Input: part model. Units: mm. Frame: model coordinates. A direction names the side the tool comes from. Coordinates: 2 decimals unless noted, no trailing zeros. Loops run counter-clockwise (first coordinate to the right, second up) from the corner with the lowest first, then second, coordinate; pieces in that order, holes last. Notation, with made-up numbers: (6, 15.5) -> (57, 15.5) arc R33 ccw to (57, 47.5) -> close; hole circle Ø1 at (69, 43). An arc over 180 degrees is marked (long way). Put each result on its own line as item: value. Start each with the question number.
1) Cut plane C-C (x = -8). Return the cut outline in (y, z).
2) Cut plane D-D (y = 4.25). Return the cut outline in (x, z).
3) Material intervals for L1, parallel to X at y = 3, z = 1.75; L2, parallel to Z at x = -19, y = -5.5; L3, parallel to Y at x = -22.5, z = -3.5, sorted ascending.
4) Set-up query: faces 1 (the flat face through (30, 0, 0)), 2 (the cylindrical face through (28, -3, 0)), 3 (the flat face through (-25, 3, 1)). Return all of +Z, -Z, +X, -X, +Y, -Y with unobstructed straight access to the full face (end or side cutting, diameter ignored); none if empty.
5) Cut plane A-A (z = 0). Return the cut outline in (x, y), plus the area to 3 significant figures.
Autodesk Inventor part; units mm, degrees
ref_plane "YZ Plane" through (0, 0, 0) normal (1, 0, 0) x (0, 1, 0)
ref_plane "XZ Plane" through (0, 0, 0) normal (0, 1, 0) x (-1, 0, 0)
ref_plane "XY Plane" through (0, 0, 0) normal (0, 0, 1) x (1, 0, 0)
sketch "Sketch1" plane through (0, 0, 0) normal (0, 0, 1) x (1, 0, 0)
  line L0 (0, 0) -> (0, 6)
  line L1 (0, 6) -> (25, 6)
  line L2 (25, 6) -> (25, 3)
  line L3 (25, 3) -> (30, 3)
  line L4 (30, 3) -> (30, 0)
  line L5 (30, 0) -> (0, 0)
  dimension "d0" = 6
  dimension "d1" = 3
  dimension "d2" = 5
  dimension "d3" = 25
revolve "Revolution1" add sketch "Sketch1" angle 360 about axis through (30, 0, 0) along (-1, 0, 0)
mirror "Mirror1" about plane through (0, 3, 0) normal (-1, 0, 0) of "Revolution1"
properties part number "Roller"
Results found:
1. outline: circle Ø12 at (0, 0)
2. outline: (-25, -4.24) -> (25, -4.24) -> (25, 4.24) -> (-25, 4.24) -> close
3. L1: x = -25 to 25
3. L2: z = -2.4 to 2.4
3. L3: y = -4.87 to 4.87
4. face 1: +Z, -Z, +X, +Y, -Y
4. face 2: +X
4. face 3: -X
5. outline: (-30, -3) -> (-25, -3) -> (-25, -6) -> (25, -6) -> (25, -3) -> (30, -3) -> (30, 3) -> (25, 3) -> (25, 6) -> (-25, 6) -> (-25, 3) -> (-30, 3) -> close
5. area: 660 mm2
